from build123d import *

# Parameters (mm, degrees)
SKETCH_1_R      = 2.5
EXTRUDE_1_DEPTH = 4
SKETCH_1_32_R   = 2.5
SKETCH_1_32_R_2 = 1.5
EXTRUDE_2_DEPTH = 1.75
SKETCH_1_33_R   = 2.5
SKETCH_1_33_R_2 = 1.5
EXTRUDE_3_DEPTH = 1.75


with BuildPart() as part:
    # Sketch 1 → Extrude 1 (new body)
    with BuildSketch(Plane(origin=(0, 0, 0), x_dir=(1, 0, 0), z_dir=(0, 1, 0))):
        with BuildLine():
            Line((-174.840079727, 131.119726246), (-199.840079727, 131.119726246))
            Line((-199.840079727, 131.119726246), (-224.840079727, 131.119726246))
            ThreePointArc((-224.840079727, 131.119726246), (-228.375613633, 129.655260152), (-229.840079727, 126.119726246))
            Line((-229.840079727, 126.119726246), (-229.840079727, 16.119726246))
            ThreePointArc((-229.840079727, 16.119726246), (-228.375613633, 12.58419234), (-224.840079727, 11.119726246))
            Line((-224.840079727, 11.119726246), (-199.840079727, 11.119726246))
            Line((-199.840079727, 11.119726246), (-174.840079727, 11.119726246))
            ThreePointArc((-174.840079727, 11.119726246), (-171.304545821, 12.58419234), (-169.840079727, 16.119726246))
            Line((-169.840079727, 16.119726246), (-169.840079727, 126.119726246))
            ThreePointArc((-169.840079727, 126.119726246), (-171.304545821, 129.655260152), (-174.840079727, 131.119726246))
        make_face()
        with Locations(Location((-214.840082087, 21.119726246, 0), (0, 0, 270))):
            Circle(SKETCH_1_R, mode=Mode.SUBTRACT)
        with BuildLine():
            ThreePointArc((-192.840079727, 46.119726246), (-190.718759384, 45.241046589), (-189.840079727, 43.119726246))
            Line((-189.840079727, 43.119726246), (-189.840079727, 24.119726246))
            ThreePointArc((-189.840079727, 24.119726246), (-190.718759384, 21.998405902), (-192.840079727, 21.119726246))
            Line((-192.840079727, 21.119726246), (-206.840082087, 21.119726246))
            ThreePointArc((-206.840082087, 21.119726246), (-208.961402431, 21.998405902), (-209.840082087, 24.119726246))
            Line((-209.840082087, 24.119726246), (-209.840082087, 43.119726246))
            ThreePointArc((-209.840082087, 43.119726246), (-208.961402431, 45.241046589), (-206.840082087, 46.119726246))
            Line((-206.840082087, 46.119726246), (-192.840079727, 46.119726246))
        make_face(mode=Mode.SUBTRACT)
        with Locations(Location((-214.840082087, 46.119726246, 0), (0, 0, 270))):
            Circle(SKETCH_1_R, mode=Mode.SUBTRACT)
        with Locations(Location((-184.840079727, 21.119726246, 0), (0, 0, 270))):
            Circle(SKETCH_1_R, mode=Mode.SUBTRACT)
        with BuildLine():
            ThreePointArc((-206.840082087, 56.119726246), (-208.961402431, 56.998405902), (-209.840082087, 59.119726246))
            Line((-209.840082087, 59.119726246), (-209.840082087, 83.119726246))
            ThreePointArc((-209.840082087, 83.119726246), (-208.961402431, 85.241046589), (-206.840082087, 86.119726246))
            Line((-206.840082087, 86.119726246), (-192.818063372, 86.119726246))
            ThreePointArc((-192.818063372, 86.119726246), (-190.704569987, 85.248844775), (-189.818144754, 83.141823385))
            Line((-189.818144754, 83.141823385), (-189.729591033, 71.119726246))
            Line((-189.729591033, 71.119726246), (-189.818144754, 59.097629106))
            ThreePointArc((-189.818144754, 59.097629106), (-190.704569987, 56.990607717), (-192.818063372, 56.119726246))
            Line((-192.818063372, 56.119726246), (-206.840082087, 56.119726246))
        make_face(mode=Mode.SUBTRACT)
        with Locations(Location((-184.840079727, 46.119726246, 0), (0, 0, 270))):
            Circle(SKETCH_1_R, mode=Mode.SUBTRACT)
        with Locations(Location((-214.840082087, 96.119726246, 0), (0, 0, 270))):
            Circle(SKETCH_1_R, mode=Mode.SUBTRACT)
        with Locations(Location((-214.840082087, 121.119726246, 0), (0, 0, 270))):
            Circle(SKETCH_1_R, mode=Mode.SUBTRACT)
        with BuildLine():
            Line((-192.840079727, 96.119726246), (-206.840082087, 96.119726246))
            ThreePointArc((-206.840082087, 96.119726246), (-208.961402431, 96.998405902), (-209.840082087, 99.119726246))
            Line((-209.840082087, 99.119726246), (-209.840082087, 118.119726246))
            ThreePointArc((-209.840082087, 118.119726246), (-208.961402431, 120.241046589), (-206.840082087, 121.119726246))
            Line((-206.840082087, 121.119726246), (-192.840079727, 121.119726246))
            ThreePointArc((-192.840079727, 121.119726246), (-190.718759384, 120.241046589), (-189.840079727, 118.119726246))
            Line((-189.840079727, 118.119726246), (-189.840079727, 99.119726246))
            ThreePointArc((-189.840079727, 99.119726246), (-190.718759384, 96.998405902), (-192.840079727, 96.119726246))
        make_face(mode=Mode.SUBTRACT)
        with Locations(Location((-184.840079727, 96.119726246, 0), (0, 0, 270))):
            Circle(SKETCH_1_R, mode=Mode.SUBTRACT)
        with Locations(Location((-184.840079727, 121.119726246, 0), (0, 0, 270))):
            Circle(SKETCH_1_R, mode=Mode.SUBTRACT)
    extrude(amount=EXTRUDE_1_DEPTH)

    # Sketch 1_32 → Extrude 2 (add)
    # profile 1 of 4: a face of its own
    with BuildSketch(Plane(origin=(0, 0, 0), x_dir=(1, 0, 0), z_dir=(0, 1, 0))):
        with Locations(Location((-214.840082087, 96.119726246, 0), (0, 0, 270))):
            Circle(SKETCH_1_32_R)
        with Locations(Location((-214.840082087, 96.119726246, 0), (0, 0, 270))):
            Circle(SKETCH_1_32_R_2, mode=Mode.SUBTRACT)
    # profile 2 of 4: a face of its own
    with BuildSketch(Plane(origin=(0, 0, 0), x_dir=(1, 0, 0), z_dir=(0, 1, 0))):
        with Locations(Location((-184.840079727, 96.119726246, 0), (0, 0, 270))):
            Circle(SKETCH_1_32_R)
        with Locations(Location((-184.840079727, 96.119726246, 0), (0, 0, 270))):
            Circle(SKETCH_1_32_R_2, mode=Mode.SUBTRACT)
    # profile 3 of 4: a face of its own
    with BuildSketch(Plane(origin=(0, 0, 0), x_dir=(1, 0, 0), z_dir=(0, 1, 0))):
        with Locations(Location((-184.840079727, 121.119726246, 0), (0, 0, 270))):
            Circle(SKETCH_1_32_R)
        with Locations(Location((-184.840079727, 121.119726246, 0), (0, 0, 270))):
            Circle(SKETCH_1_32_R_2, mode=Mode.SUBTRACT)
    # profile 4 of 4: a face of its own
    with BuildSketch(Plane(origin=(0, 0, 0), x_dir=(1, 0, 0), z_dir=(0, 1, 0))):
        with Locations(Location((-214.840082087, 121.119726246, 0), (0, 0, 270))):
            Circle(SKETCH_1_32_R)
        with Locations(Location((-214.840082087, 121.119726246, 0), (0, 0, 270))):
            Circle(SKETCH_1_32_R_2, mode=Mode.SUBTRACT)
    extrude(amount=EXTRUDE_2_DEPTH)

    # Sketch 1_33 → Extrude 3 (add)
    # profile 1 of 4: a face of its own
    with BuildSketch(Plane(origin=(0, 0, 0), x_dir=(1, 0, 0), z_dir=(0, 1, 0))):
        with Locations(Location((-214.840082087, 46.119726246, 0), (0, 0, 270))):
            Circle(SKETCH_1_33_R)
        with Locations(Location((-214.840082087, 46.119726246, 0), (0, 0, 270))):
            Circle(SKETCH_1_33_R_2, mode=Mode.SUBTRACT)
    # profile 2 of 4: a face of its own
    with BuildSketch(Plane(origin=(0, 0, 0), x_dir=(1, 0, 0), z_dir=(0, 1, 0))):
        with Locations(Location((-184.840079727, 46.119726246, 0), (0, 0, 270))):
            Circle(SKETCH_1_33_R)
        with Locations(Location((-184.840079727, 46.119726246, 0), (0, 0, 270))):
            Circle(SKETCH_1_33_R_2, mode=Mode.SUBTRACT)
    # profile 3 of 4: a face of its own
    with BuildSketch(Plane(origin=(0, 0, 0), x_dir=(1, 0, 0), z_dir=(0, 1, 0))):
        with Locations(Location((-214.840082087, 21.119726246, 0), (0, 0, 270))):
            Circle(SKETCH_1_33_R)
        with Locations(Location((-214.840082087, 21.119726246, 0), (0, 0, 270))):
            Circle(SKETCH_1_33_R_2, mode=Mode.SUBTRACT)
    # profile 4 of 4: a face of its own
    with BuildSketch(Plane(origin=(0, 0, 0), x_dir=(1, 0, 0), z_dir=(0, 1, 0))):
        with Locations(Location((-184.840079727, 21.119726246, 0), (0, 0, 270))):
            Circle(SKETCH_1_33_R)
        with Locations(Location((-184.840079727, 21.119726246, 0), (0, 0, 270))):
            Circle(SKETCH_1_33_R_2, mode=Mode.SUBTRACT)
    extrude(amount=EXTRUDE_3_DEPTH)


solid = part.part
Can you work these out from the model? Positions are in its coordinate system, mm. A direction names the side the tool comes from. Give positions to 0.01 mm unless a question says otherwise; leave off trailing zeros. Loops run counter-clockwise (first coordinate to the right, second up) from the corner with the lowest first, then second, coordinate; pieces in that order, holes last. Notation, with made-up numbers: (82.5, 89.25) - (108.5, 89.25) arc R8 ccw to (108.5, 93.25) - close; hole circle Ø5 at (-1, 3). An arc over 180 degrees is marked (long way). Answer as a JSON object with one key per item and string values.
Q1. Imagine slicing it at B-B on x = -194.5. Write out the boundary of the cut face in (y, z), plus the area to 3 significant figures.
Geometry says:
{"outline": "(0, -131.12) - (4, -131.12) - (4, -121.12) - (0, -121.12) - close; (0, -96.12) - (4, -96.12) - (4, -86.12) - (0, -86.12) - close; (0, -56.12) - (4, -56.12) - (4, -46.12) - (0, -46.12) - close; (0, -21.12) - (4, -21.12) - (4, -11.12) - (0, -11.12) - close", "area": "160 mm²"}
Q2. Imagine slicing it at A-A on z = -116.5. Write out the boundary of the cut face in (x, y), plus the area to 3 significant figures.
Geometry says:
{"outline": "(-229.84, 0) - (-209.84, 0) - (-209.84, 4) - (-229.84, 4) - close; (-189.84, 0) - (-169.84, 0) - (-169.84, 4) - (-189.84, 4) - close", "area": "160 mm²"}
Q3. If we mould it in two halves opening along Z, with no side actions, what happens to faces 4 (the flat face through (-200, 2, -121.12)), 5 (the cylindrical face through (-171.34, 1.97, -12.55)), 6 (the flat face through (-199, 2, -131.12))? For each: pulls with the +Z half, pulls with the -Z half, needs draft (parallel to the pull), parting line crosses it, or undercut.
Geometry says:
{"face 4": "undercut", "face 5": "pulls with the +Z half", "face 6": "pulls with the -Z half"}
Q4. Imagine slicing it at D-D on z = -78. Write out the boundary of the cut face in (x, y).
Geometry says:
{"outline": "(-229.84, 0) - (-209.84, 0) - (-209.84, 4) - (-229.84, 4) - close; (-189.78, 0) - (-169.84, 0) - (-169.84, 4) - (-189.78, 4) - close"}
Q5. Will these pins go through, and if not, where does the flat tip stop? P1, Ø5, axis at x = -214.84, z = -121.12, coming from the -Y side; P2, Ø3.5, axis at x = -184.84, z = -46.12, coming from the +Y side.
Geometry says:
{"P1": "y = 0", "P2": "y = 1.75"}
Q6. If I drill on L1, parallel to Z at x = -205, y = 3.75; L2, parallel to Z at x = -185, y = 1.25; L3, parallel to Z at x = -183.5, y = 3.6, over which ranges is the centre line in solid material (lowest first)?
Geometry says:
{"L1": "-131.12 to -121.12, -96.12 to -86.12, -56.12 to -46.12, -21.12 to -11.12", "L2": "-131.12 to -122.61, -119.63 to -97.61, -94.63 to -47.61, -44.63 to -22.61, -19.63 to -11.12", "L3": "-131.12 to -123.23, -119.01 to -98.23, -94.01 to -48.23, -44.01 to -23.23, -19.01 to -11.12"}
Q7. Which directions (+Z, -Z, +X, -X, +Y, -Y) give clear straight access to the entire face, cutting with the end or side of a thin tool? Please do faces 1 (the flat face through (-229.84, 2, -72)), 2 (the flat face through (-186.5, 1.75, -96.2)), 3 (the cylindrical face through (-190.681, 1.972, -57.014)).
Geometry says:
{"face 1": "+Z, -Z, -X, +Y, -Y", "face 2": "+Y", "face 3": "+Y, -Y"}
Q8. Imagine slicing it at C-C on y = 2.35. Give the number of separate pieces and of enclosed holes in the cut face, plus the area to 3 significant figures.
Geometry says:
{"separate pieces": "1", "enclosed holes": "11", "area": "5,440 mm²"}
